```python
from build123d import *

# Parameters (mm, degrees)
BOSS_EXTRUDE1_DEPTH = 10
BOSS_EXTRUDE2_DEPTH = 13
SKETCH4_W           = 151.79281634
SKETCH4_H           = 122.98522628
BOSS_EXTRUDE3_DEPTH = 10
SKETCH5_R           = 2.8
CUT_EXTRUDE1_DEPTH  = 101.99281634
FILLET1_R           = 6.35


with BuildPart() as part:
    # Sketch1 → Boss-Extrude1 (new body)
    with BuildSketch(Plane.XY):
        Polygon((-24.634, 0), (-24.634, 13), (70.616, 67.99261314), (70.616, -54.99261314), align=None)
    extrude(amount=BOSS_EXTRUDE1_DEPTH)

    # Sketch3 → Boss-Extrude2 (add)
    with BuildSketch(Plane(origin=(0, 13, 0), x_dir=(1, 0, 0), z_dir=(0, 1, 0))):
        Polygon((70.616, -50.19281634), (70.616, -10), (1, -10), align=None)
    extrude(amount=-BOSS_EXTRUDE2_DEPTH)

    # Sketch4 → Boss-Extrude3 (add)
    with BuildSketch(Plane(origin=(70.616, 0, 0), x_dir=(0, 0, -1), z_dir=(1, 0, 0))):
        with Locations((-25.09640817, 6.5)):
            Rectangle(SKETCH4_W, SKETCH4_H)
    extrude(amount=BOSS_EXTRUDE3_DEPTH)

    # Sketch5 → Cut-Extrude1 (cut, through all)
    with BuildSketch(Plane(origin=(0, 0, 0), x_dir=(-1, 0, 0), z_dir=(0, 0, -1))):
        with Locations((5.067, 6.5)):
            Circle(SKETCH5_R)
        with Locations((19.567, 6.5)):
            Circle(SKETCH5_R)
    extrude(amount=-CUT_EXTRUDE1_DEPTH, mode=Mode.SUBTRACT)

    # Fillet1
    fillet1_edges = [part.edges().sort_by_distance(p)[0] for p in [
        (70.616, 40.49630657, 10),
        (70.616, 6.5, 50.19281634),
        (35.808, 13, 10),
        (70.616, 13, 30.09640817),
        (35.808, 0, 10),
        (70.616, 0, 30.09640817),
        (70.616, -27.49630657, 10),
        (70.616, 6.5, 0),
    ]]
    fillet(fillet1_edges, radius=FILLET1_R)


solid = part.part
```
The listing builds one solid part. Answer for the finished solid, in the listing's coordinates (mm). A direction names the side the tool comes from. Coordinates: 2 decimals unless noted, no trailing zeros. Order: outer loops, then holes, each group sorted by start corner. A loop starts at its lowest first (then second) coordinate and runs counter-clockwise, first axis right, second up. Notation, with made-up numbers: M -16,79 L 6,79 A33 cw 6,118 Z; hole C 87.25,21 d10. An arc over 180 degrees is marked long. Answer as a JSON object with one key per item and string values. Group by question number.
1. Section A-A on y = 6.5 is taken. Write down the section's boundary in (x, z), then the cut area to 3 significant figures.
2. Straight lines are drawn through the part: line 1 (X direction, y = 6, z = 6); line 2 (X direction, y = -39.5, z = 17); line 3 (Z direction, x = 49.5, y = 28). For each, find the intervals that lie inside material, in ascending order.
3. Determine the mould class of faces 4 (the cylindrical face through (-6.359, 4.016, 4.93)), 5 (the flat face through (49, 13, 25)), 6 (the cylindrical face through (68.805, 43.331, 11.91)) for opening direction X: released by +X, released by -X, zero draft, split by the parting line, or undercut.
4. Flat-ended cylindrical pins translate along their axes: P1, Ø5, axis at x = 57, y = -34, coming from the +Z side; P2, Ø12, axis at y = 48.5, z = 17.5, coming from the -X side; P3, Ø1.5, axis at x = 37, y = -8, coming from the -Z side. Find the tip coordinate at first contact, or state that the pin passes through.
5. Section B-B on x = 50 is taken. Write down the section's boundary in (y, z), then the cut area to 3 significant figures.
6. Section D-D on z = 76.5 is taken. Write down the section's boundary in (x, y).
7. Section C-C on y = 57 is taken. Write down the section's boundary in (x, z), then the cut area to 3 significant figures.
8. A tool of negligible diameter and unlimited length cuts with its end or side. For faces 1 (the cylindrical face through (68.805, -31.012, 11.91)), 2 (the flat face through (30, 7, 0)), 3 (the cylindrical face through (68.805, 14.91, 34.842)), from which of +Z, -Z, +X, -X, +Y, -Y can it reach the whole face along a straight path? Write none if from no direction.
Values follow:
{
 "1": {"outline": "M -24.63,0 L -22.37,0 L -22.37,10 L -24.63,10 Z; M -16.77,0 L -7.87,0 L -7.87,10 L -16.77,10 Z; M -2.27,0 L 64.27,0 A6.35 cw 70.62,-6.35 L 70.62,-50.8 L 80.62,-50.8 L 80.62,100.99 L 70.62,100.99 L 70.62,53.86 A6.35 cw 67.44,48.36 L 1,10 L -2.27,10 Z", "area": "3,770 mm2"},
 "2": {"line 1": "-24.63 to -22.32, -16.81 to -7.82, -2.31 to 80.62", "line 2": "70.62 to 80.62", "line 3": "0 to 10"},
 "3": {"face 4": "undercut", "face 5": "zero draft", "face 6": "released by -X"},
 "4": {"P1": "z = 10", "P2": "x = 68.36", "P3": "z = 0"},
 "5": {"outline": "M -43.09,0 L 56.09,0 L 56.09,10 L 19.35,10 A6.35 cw 13,16.35 L 13,38.29 L 0,38.29 L 0,16.35 A6.35 cw -6.35,10 L -43.09,10 Z", "area": "1,380 mm2"},
 "6": {"outline": "M 70.62,-54.99 L 80.62,-54.99 L 80.62,67.99 L 70.62,67.99 Z"},
 "7": {"outline": "M 51.58,0 L 64.27,0 A6.35 cw 70.62,-6.35 L 70.62,-50.8 L 80.62,-50.8 L 80.62,100.99 L 70.62,100.99 L 70.62,16.35 A6.35 cw 64.27,10 L 51.58,10 Z", "area": "1,730 mm2"},
 "8": {"face 1": "+Z, -X, -Y", "face 2": "-Z, -X, +Y, -Y", "face 3": "+Z, -X, +Y"}
}
